Input: dimensioned drawing with shaded views. Units: mm. Origin: part minimum x, y, z. A direction names the side the tool comes from. Coordinates: 2 decimals unless noted, no trailing zeros. Loops run counter-clockwise (first coordinate to the right, second up) from the corner with the lowest first, then second, coordinate; pieces in that order, holes last.
Item 1: Section C-C on x = 1.9. Return loops of the section in (y, z).
Item 2: Contact query for flat-ended pins moving along their axis: P1, Ø2.5, axis at x = 39.1, y = 11, coming from the +Z side; P2, Ø3.5, axis at x = 39.1, y = 2, coming from the -Z side; P3, Ø4, axis at y = 5, z = 1.5, coming from the -X side; P4, Ø2, axis at x = 35, z = 4, coming from the -Y side. Output: stop coordinate, or through.
Item 3: Reachability of the marked faces 5, 6 and 7 from +Z, -Z, +X, -X, +Y, -Y: full face, straight path, thin tool, end or side. Return the list, or none.
Item 4: Section D-D on y = 9. Return loops of the section in (x, z), and give its area (3 significant figures).
Item 5: Pull-direction query (X, two-part tool) for the marked faces 1, 2, 3 and 4; classes: released by +X, released by -X, zero draft, split by the parting line, or undercut.
Item 6: Section B-B on z = 8.25. Return loops of the section in (x, y).
Item 7: Section A-A on y = 11. Return loops of the section in (x, z), and give its area (3 significant figures).
Item 8: Ray query, line 1 along Y through (x, z) = (1.9, 9.1); line 2 along X through (y, z) = (11.5, 9.25); line 3 along Z through (x, y) = (10, 1.25). Return the intervals inside material, ascending.
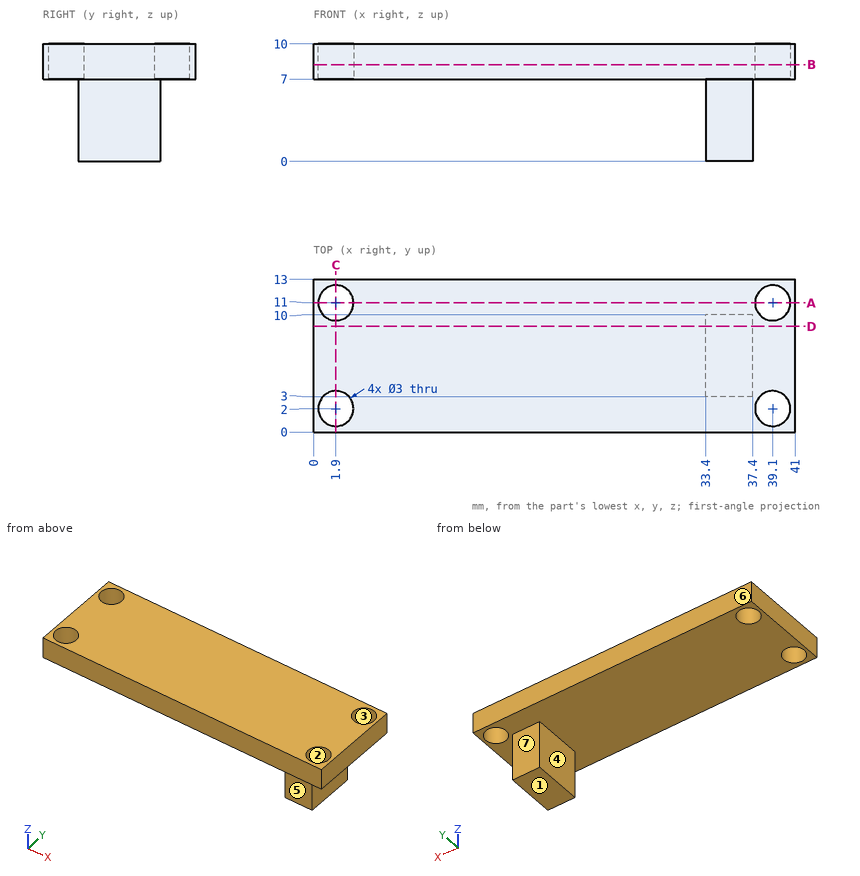
Results found:
1. outline: (0, 7) - (0.5, 7) - (0.5, 10) - (0, 10) - close; (3.5, 7) - (9.5, 7) - (9.5, 10) - (3.5, 10) - close; (12.5, 7) - (13, 7) - (13, 10) - (12.5, 10) - close
2. P1: passes through
2. P2: stops at z = 7
2. P3: stops at x = 33.4
2. P4: stops at y = 3
3. face 5: -Z, +X, -X, -Y
3. face 6: +Z, -Z, +X, -X, +Y
3. face 7: -Z, +X, -X, +Y
4. outline: (0, 7) - (33.4, 7) - (33.4, 0) - (37.4, 0) - (37.4, 7) - (41, 7) - (41, 10) - (0, 10) - close
4. area: 151 mm2
5. face 1: zero draft
5. face 2: undercut
5. face 3: undercut
5. face 4: released by -X
6. outline: (0, 0) - (41, 0) - (41, 13) - (0, 13) - close; hole circle Ø3 at (1.9, 2); hole circle Ø3 at (1.9, 11); hole circle Ø3 at (39.1, 2); hole circle Ø3 at (39.1, 11)
7. outline: (0, 7) - (0.4, 7) - (0.4, 10) - (0, 10) - close; (3.4, 7) - (37.6, 7) - (37.6, 10) - (3.4, 10) - close; (40.6, 7) - (41, 7) - (41, 10) - (40.6, 10) - close
7. area: 105 mm2
8. line 1: y = 0 to 0.5, 3.5 to 9.5, 12.5 to 13
8. line 2: x = 0 to 0.49, 3.31 to 37.69, 40.51 to 41
8. line 3: z = 7 to 10
